Drawing for the job (mm, zero at the part's lowest x, y, z). Give positions to 0.01 mm unless a question says otherwise; leave off trailing zeros. Order: outer loops, then holes, each group sorted by start corner. A loop starts at its lowest first (then second) coordinate and runs counter-clockwise, first axis right, second up. Notation, with made-up numbers: (-2.75, 12.25) - (55.25, 12.25) arc R33 cw to (55.25, 48.25) - close; hole circle Ø9 at (-40, 60.5). An arc over 180 degrees is marked (long way). One line per item, written item: value.
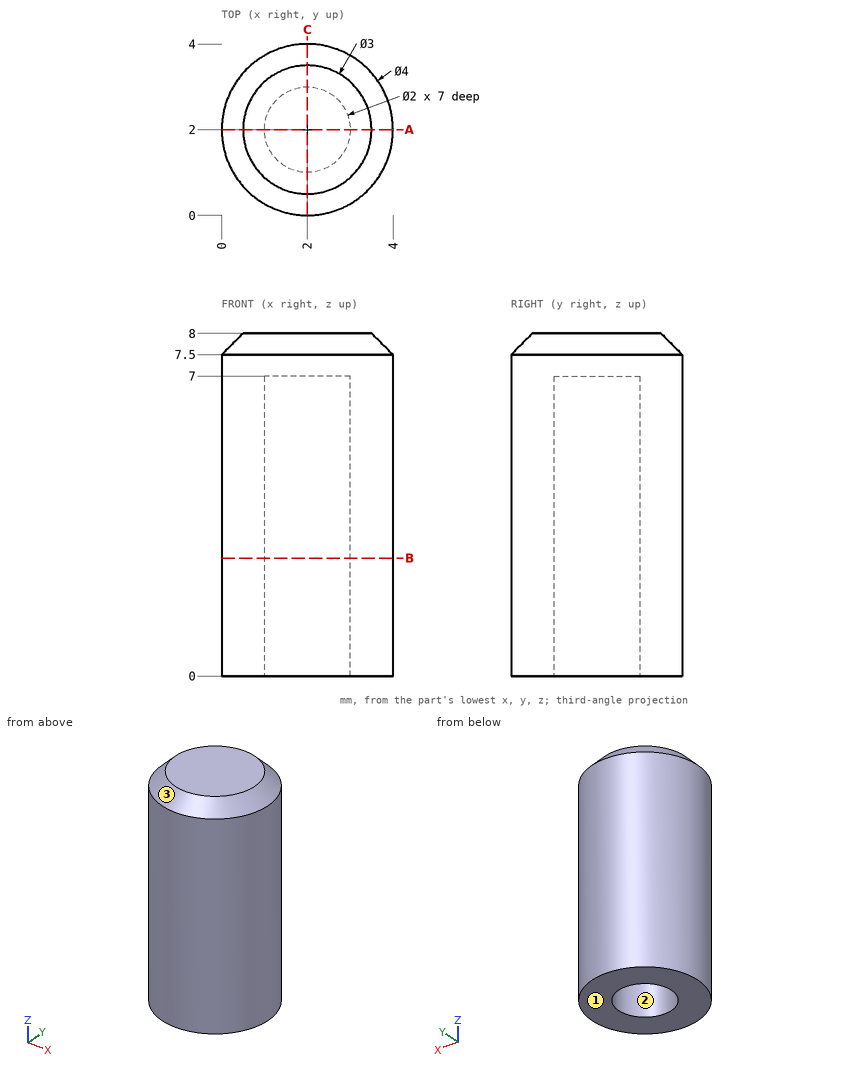
(1) Pull direction Y, two halves, no side cores. Call the marked faces 1, 2 and 3: +Y half, -Y half, draft (parallel to the pull), parting line (faces both ways), or undercut.
Completed:
face 1: draft
face 2: undercut
face 3: parting line
(2) Slice it at A-A, the plane y = 2. Give the cut face in (x, z), and give its area (4 significant figures).
Completed:
outline: (0, 0) - (1, 0) - (1, 7) - (3, 7) - (3, 0) - (4, 0) - (4, 7.5) - (3.5, 8) - (0.5, 8) - (0, 7.5) - close
area: 17.75 mm²
(3) Slice it at B-B, the plane z = 2.75. Give the cut face in (x, y), and give its area (3 significant figures).
Completed:
outline: circle Ø4 at (2, 2); hole circle Ø2 at (2, 2)
area: 9.42 mm²
(4) Drill centre lines: line 1 (Y direction, x = 2, z = 3.25); line 2 (Z direction, x = 1.65, y = 1.25); line 3 (X direction, y = 1.65, z = 2.75). Where is each one in solid material? Low to high.
Completed:
line 1: 0 to 1, 3 to 4
line 2: 7 to 8
line 3: 0.03 to 1.06, 2.94 to 3.97
(5) Pin check, flat tips, straight feed: P1, Ø1, axis at x = 2, y = 2, coming from the -Z side; P2, Ø1.5, axis at x = 3.5, z = 1.5, coming from the -Y side; P3, Ø1, axis at y = 1, z = 5, coming from the -X side. Stop position of each tip, or through.
Completed:
P1: z = 7
P2: y = 0.15
P3: x = 0.06
